Read the model definition and answer for the solid it produces. Units are mm, in the model's axes. Face numbers are marked on the shaded views. A direction names the side the tool comes from. Give positions to 0.01 mm unless a question says otherwise; leave off trailing zeros. Loops run counter-clockwise (first coordinate to the right, second up) from the corner with the lowest first, then second, coordinate; pieces in that order, holes last. Notation, with made-up numbers: (-7, -33) - (36, -33) arc R11 cw to (36, -23) - close; hole circle Ø1 at (72, -11.75). An arc over 180 degrees is marked (long way). Write each question's results on one line, items separated by ' | '. Start each with the question number.
Q1. The part is cut by section B-B, the plane z = 13.75. Write down the section's boundary in (x, y), plus the area to 3 significant figures.
Q2. Given pin 1 (5 mm diameter, centred on y = 12, z = 10.5, fed in from -X); pin 2 (8 mm diameter, centred on y = 20.5, z = 4, fed in from -X); pin 3 (2 mm diameter, centred on x = 18.5, z = 7.5, fed in from +Y); pin 4 (10.5 mm diameter, centred on y = 18, z = 12.5, fed in from +X), each flat-ended and moving along its own axis, determine where each tip first touches the part or whether it passes through.
Q3. The part is cut by section C-C, the plane x = 34.5. Write down the section's boundary in (y, z).
Q4. Find the intervals of material crossed by line 1 (Y direction, x = 30.5, z = 12.5); line 2 (Y direction, x = 34.5, z = 13.65); line 3 (X direction, y = 12, z = 11.25), in increasing order. Write a range as from..to.
Q5. The part is cut by section A-A, the plane y = 12.75. Write down the section's boundary in (x, z), plus the area to 3 significant figures.
Q6. The part is cut by section D-D, the plane z = 9. Write down the section's boundary in (x, y), plus the area to 4 significant figures.
Q7. Determine the mould class of the marked faces 4, 5 and 6 for opening direction Y: +Y half, -Y half, draft (parallel to the pull), parting line (faces both ways), or undercut.
Q8. For the marked faces 1, 2 and 3, determine the directions among +Z, -Z, +X, -X, +Y, -Y from which every point of the face is accessible in a straight line to the end or side of a thin tool.
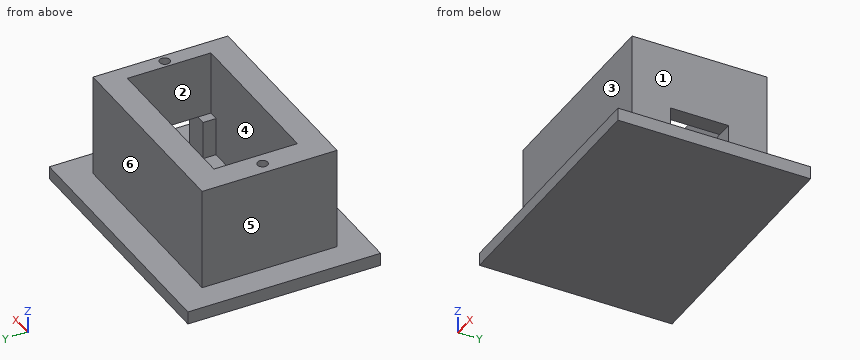
```python
from build123d import *

# Parameters (mm, degrees)
BOX_W         = 40
BOX_H         = 30
BOX_DEPTH     = 2
PAD_DEPTH     = 6
SKETCH001_W   = 31.5
SKETCH001_H   = 21
SKETCH001_W_2 = 25
SKETCH001_H_2 = 13
PAD001_DEPTH  = 10
SKETCH002_R   = 0.8
POCKET_DEPTH  = 6


with BuildPart() as part:
    # Box → Box (new body)
    with BuildSketch(Plane.XY):
        with Locations((20, 15)):
            Rectangle(BOX_W, BOX_H)
    extrude(amount=BOX_DEPTH)

    # Sketch (on Face6 of BaseFeature) → Pad (new body)
    with BuildSketch(Plane.XY.offset(2)):
        Polygon((35.75, 19.5), (35.75, 25.5), (4.25, 25.5), (4.25, 4.5), (35.75, 4.5), (35.75, 10.5), (31.75, 10.5), (31.75, 8.5), (8.25, 8.5), (8.25, 21.5), (31.75, 21.5), (31.75, 19.5), align=None)
    extrude(amount=PAD_DEPTH)

    # Sketch001 (on Face19 of Pad) → Pad001 (join)
    with BuildSketch(Plane.XY.offset(8)):
        with Locations((20, 15)):
            Rectangle(SKETCH001_W, SKETCH001_H)
        with Locations((20.75, 15)):
            Rectangle(SKETCH001_W_2, SKETCH001_H_2, mode=Mode.SUBTRACT)
    extrude(amount=PAD001_DEPTH)

    # Sketch002 (on Face29 of Pad001) → Pocket (cut)
    with BuildSketch(Plane.XY.offset(18)):
        with Locations((6.25, 15)):
            Circle(SKETCH002_R)
        with Locations((34.5, 15)):
            Circle(SKETCH002_R)
    extrude(amount=-POCKET_DEPTH, mode=Mode.SUBTRACT)


solid = part.part
```
Check sheet entries:
1) outline: (4.25, 4.5) - (35.75, 4.5) - (35.75, 25.5) - (4.25, 25.5) - close; hole circle Ø1.6 at (6.25, 15); hole (8.25, 8.5) - (33.25, 8.5) - (33.25, 21.5) - (8.25, 21.5) - close; hole circle Ø1.6 at (34.5, 15) | area: 332 mm^2
2) pin 1: stops at x = 4.25 | pin 2: stops at x = 0 | pin 3: stops at y = 25.5 | pin 4: stops at x = 35.75
3) outline: (0, 0) - (30, 0) - (30, 2) - (25.5, 2) - (25.5, 18) - (15.8, 18) - (15.8, 12) - (14.2, 12) - (14.2, 18) - (4.5, 18) - (4.5, 2) - (0, 2) - close; hole (10.5, 2) - (19.5, 2) - (19.5, 8) - (10.5, 8) - close
4) line 1: y = 4.5..8.5, 21.5..25.5 | line 2: y = 4.5..14.2, 15.8..25.5 | line 3: x = 4.25..8.25, 33.25..35.75
5) outline: (0, 0) - (40, 0) - (40, 2) - (8.25, 2) - (8.25, 18) - (4.25, 18) - (4.25, 2) - (0, 2) - close; (33.25, 8) - (35.75, 8) - (35.75, 18) - (33.25, 18) - close | area: 169 mm^2
6) outline: (4.25, 4.5) - (35.75, 4.5) - (35.75, 25.5) - (4.25, 25.5) - close; hole (8.25, 8.5) - (33.25, 8.5) - (33.25, 21.5) - (8.25, 21.5) - close | area: 336.5 mm^2
7) face 4: undercut | face 5: draft | face 6: +Y half
8) face 1: +Z, +X, +Y, -Y | face 2: +Z | face 3: +Z, +X, -X, -Y
